Check sheet for the modelled part. Datum: model origin and axes. Units: mm. Face numbers are marked on the shaded views. Coordinates: 2 decimals unless noted, no trailing zeros. Write each loop counter-clockwise with the first axis right and the second up, starting at its lowest first coordinate (ties: lowest second). Pieces come first, ordered by that corner, then holes. Notation, with made-up numbers: (59.25, 89) - (70.25, 89) arc R17 cw to (70.25, 93) - close; hole circle Ø10 at (83.5, 89.5). An arc over 180 degrees is marked (long way). Write each question's results on one line, items separated by ' | '.
from build123d import *

# Parameters (mm, degrees)
SKETCH1_R           = 1.075
SKETCH1_R_2         = 3.5
BOSS_EXTRUDE1_DEPTH = 2.15
SKETCH2_R           = 1.075
BOSS_EXTRUDE2_DEPTH = 2.5


with BuildPart() as part:
    # Sketch1 → Boss-Extrude1 (new body)
    with BuildSketch(Plane(origin=(0, 0, 0), x_dir=(1, 0, 0), z_dir=(0, 1, 0))):
        with BuildLine():
            Line((-30, 19.443650814), (-30, -19.443650814))
            ThreePointArc((-30, -19.443650814), (-30.380602337, -21.357067976), (-31.464466094, -22.97918472))
            Line((-31.464466094, -22.97918472), (-39.242640687, -30.757359313))
            ThreePointArc((-39.242640687, -30.757359313), (-39.242640687, -39.242640687), (-30.757359313, -39.242640687))
            Line((-30.757359313, -39.242640687), (-22.97918472, -31.464466094))
            ThreePointArc((-22.97918472, -31.464466094), (-21.357067976, -30.380602337), (-19.443650814, -30))
            Line((-19.443650814, -30), (19.443650814, -30))
            ThreePointArc((19.443650814, -30), (21.357067976, -30.380602337), (22.97918472, -31.464466094))
            Line((22.97918472, -31.464466094), (30.757359313, -39.242640687))
            ThreePointArc((30.757359313, -39.242640687), (39.242640687, -39.242640687), (39.242640687, -30.757359313))
            Line((39.242640687, -30.757359313), (31.464466094, -22.97918472))
            ThreePointArc((31.464466094, -22.97918472), (30.380602337, -21.357067976), (30, -19.443650814))
            Line((30, -19.443650814), (30, 19.443650814))
            ThreePointArc((30, 19.443650814), (30.380602337, 21.357067976), (31.464466094, 22.97918472))
            Line((31.464466094, 22.97918472), (39.242640687, 30.757359313))
            ThreePointArc((39.242640687, 30.757359313), (39.242640687, 39.242640687), (30.757359313, 39.242640687))
            Line((30.757359313, 39.242640687), (22.97918472, 31.464466094))
            ThreePointArc((22.97918472, 31.464466094), (21.357067976, 30.380602337), (19.443650814, 30))
            Line((19.443650814, 30), (-19.443650814, 30))
            ThreePointArc((-19.443650814, 30), (-21.357067976, 30.380602337), (-22.97918472, 31.464466094))
            Line((-22.97918472, 31.464466094), (-30.757359313, 39.242640687))
            ThreePointArc((-30.757359313, 39.242640687), (-39.242640687, 39.242640687), (-39.242640687, 30.757359313))
            Line((-39.242640687, 30.757359313), (-31.464466094, 22.97918472))
            ThreePointArc((-31.464466094, 22.97918472), (-30.380602337, 21.357067976), (-30, 19.443650814))
        make_face()
        with Locations((-24.245, 24.245)):
            Circle(SKETCH1_R, mode=Mode.SUBTRACT)
        with Locations((24.245, 24.245)):
            Circle(SKETCH1_R, mode=Mode.SUBTRACT)
        with Locations((24.245, -24.245)):
            Circle(SKETCH1_R, mode=Mode.SUBTRACT)
        with Locations((-24.245, -24.245)):
            Circle(SKETCH1_R, mode=Mode.SUBTRACT)
        with Locations((35, -35)):
            Circle(SKETCH1_R_2, mode=Mode.SUBTRACT)
        with Locations((-35, -35)):
            Circle(SKETCH1_R_2, mode=Mode.SUBTRACT)
        with Locations((-35, 35)):
            Circle(SKETCH1_R_2, mode=Mode.SUBTRACT)
        with Locations((35, 35)):
            Circle(SKETCH1_R_2, mode=Mode.SUBTRACT)
        with BuildLine():
            Line((-15, -17.5), (15, -17.5))
            ThreePointArc((15, -17.5), (16.767766953, -16.767766953), (17.5, -15))
            Line((17.5, -15), (17.5, 15))
            ThreePointArc((17.5, 15), (16.767766953, 16.767766953), (15, 17.5))
            Line((15, 17.5), (-15, 17.5))
            ThreePointArc((-15, 17.5), (-16.767766953, 16.767766953), (-17.5, 15))
            Line((-17.5, 15), (-17.5, -15))
            ThreePointArc((-17.5, -15), (-16.767766953, -16.767766953), (-15, -17.5))
        make_face(mode=Mode.SUBTRACT)
    extrude(amount=BOSS_EXTRUDE1_DEPTH)

    # Sketch2 → Boss-Extrude2 (add)
    with BuildSketch(Plane.XZ):
        with BuildLine():
            Line((27.32, -24.245), (27.32, -14.245))
            ThreePointArc((27.32, -14.245), (24.245, -11.17), (21.17, -14.245))
            Line((21.17, -14.245), (21.17, -18.67))
            ThreePointArc((21.17, -18.67), (20.437766953, -20.437766953), (18.67, -21.17))
            Line((18.67, -21.17), (14.245, -21.17))
            ThreePointArc((14.245, -21.17), (11.17, -24.245), (14.245, -27.32))
            Line((14.245, -27.32), (24.245, -27.32))
            ThreePointArc((24.245, -27.32), (26.419353352, -26.419353352), (27.32, -24.245))
        make_face()
        with Locations((24.245, -24.245)):
            Circle(SKETCH2_R, mode=Mode.SUBTRACT)
        with BuildLine():
            Line((-24.245, -27.32), (-14.245, -27.32))
            ThreePointArc((-14.245, -27.32), (-11.17, -24.245), (-14.245, -21.17))
            Line((-14.245, -21.17), (-18.67, -21.17))
            ThreePointArc((-18.67, -21.17), (-20.437766953, -20.437766953), (-21.17, -18.67))
            Line((-21.17, -18.67), (-21.17, -14.245))
            ThreePointArc((-21.17, -14.245), (-24.245, -11.17), (-27.32, -14.245))
            Line((-27.32, -14.245), (-27.32, -24.245))
            ThreePointArc((-27.32, -24.245), (-26.419353352, -26.419353352), (-24.245, -27.32))
        make_face()
        with Locations((-24.245, -24.245)):
            Circle(SKETCH2_R, mode=Mode.SUBTRACT)
        with BuildLine():
            Line((-27.32, 24.245), (-27.32, 14.245))
            ThreePointArc((-27.32, 14.245), (-24.245, 11.17), (-21.17, 14.245))
            Line((-21.17, 14.245), (-21.17, 18.67))
            ThreePointArc((-21.17, 18.67), (-20.437766953, 20.437766953), (-18.67, 21.17))
            Line((-18.67, 21.17), (-14.245, 21.17))
            ThreePointArc((-14.245, 21.17), (-11.17, 24.245), (-14.245, 27.32))
            Line((-14.245, 27.32), (-24.245, 27.32))
            ThreePointArc((-24.245, 27.32), (-26.419353352, 26.419353352), (-27.32, 24.245))
        make_face()
        with Locations((-24.245, 24.245)):
            Circle(SKETCH2_R, mode=Mode.SUBTRACT)
        with BuildLine():
            Line((24.245, 27.32), (14.245, 27.32))
            ThreePointArc((14.245, 27.32), (11.17, 24.245), (14.245, 21.17))
            Line((14.245, 21.17), (18.67, 21.17))
            ThreePointArc((18.67, 21.17), (20.437766953, 20.437766953), (21.17, 18.67))
            Line((21.17, 18.67), (21.17, 14.245))
            ThreePointArc((21.17, 14.245), (24.245, 11.17), (27.32, 14.245))
            Line((27.32, 14.245), (27.32, 24.245))
            ThreePointArc((27.32, 24.245), (26.419353352, 26.419353352), (24.245, 27.32))
        make_face()
        with Locations((24.245, 24.245)):
            Circle(SKETCH2_R, mode=Mode.SUBTRACT)
    extrude(amount=BOSS_EXTRUDE2_DEPTH)


solid = part.part
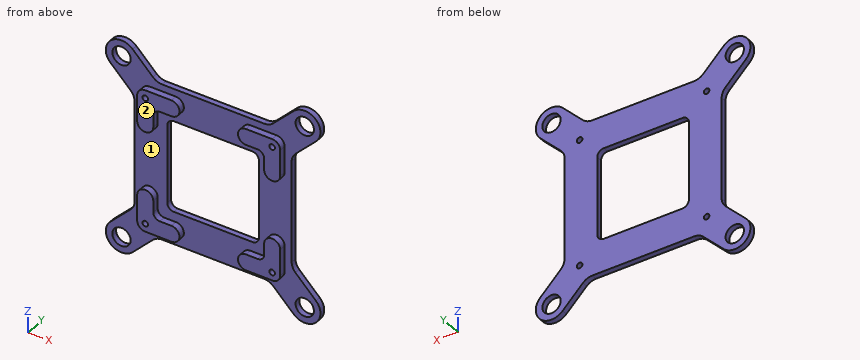
1. Sectioned sample at C-C (y = -1.5). Give the number of separate pieces and of enclosed holes in the cut face, then the cut area to 3 significant figures.
Values follow:
separate pieces: 4 | enclosed holes: 4 | area: 594 mm^2
2. Material ranges on L1, parallel to Z at x = 5, y = 1.4; L2, parallel to X at y = -1.15, z = 14; L3, parallel to Z at x = -23.5, y = -1.9, recorded low to high. Write a range as [from, to].
Values follow:
L1: z = [-30, -17.5], [17.5, 30] | L2: x = [-27.31, -21.18], [21.18, 27.31] | L3: z = [-27.32, -25.02], [-23.47, -11.26], [11.26, 23.47], [25.02, 27.32]
3. Sectioned sample at D-D (x = 36). Record the cut outline in (y, z).
Values follow:
outline: (0, -40.92) - (2.15, -40.92) - (2.15, -38.35) - (0, -38.35) - close; (0, -31.65) - (2.15, -31.65) - (2.15, -27.51) - (0, -27.51) - close; (0, 27.51) - (2.15, 27.51) - (2.15, 31.65) - (0, 31.65) - close; (0, 38.35) - (2.15, 38.35) - (2.15, 40.92) - (0, 40.92) - close
4. Draft check along X on the marked faces 1 and 2. Enter one of: pulls with the +X half, pulls with the -X half, needs draft (parallel to the pull), parting line crosses it, or undercut.
Values follow:
face 1: undercut | face 2: needs draft
5. Sectioned sample at B-B (z = 35). Record the cut outline in (x, y), then the cut area to 3 significant figures.
Values follow:
outline: (-41, 0) - (-38.5, 0) - (-38.5, 2.15) - (-41, 2.15) - close; (-31.5, 0) - (-26.51, 0) - (-26.51, 2.15) - (-31.5, 2.15) - close; (26.51, 0) - (31.5, 0) - (31.5, 2.15) - (26.51, 2.15) - close; (38.5, 0) - (41, 0) - (41, 2.15) - (38.5, 2.15) - close | area: 32.2 mm^2
6. Sectioned sample at A-A (x = 6). Record the cut outline in (y, z).
Values follow:
outline: (0, -30) - (2.15, -30) - (2.15, -17.5) - (0, -17.5) - close; (0, 17.5) - (2.15, 17.5) - (2.15, 30) - (0, 30) - close
7. Go/stop test with flat-tipped pins: pin 1 (1.2 mm diameter, centred on y = -2, z = 17.5, fed in from +X); pin 2 (1 mm diameter, centred on x = 31.5, y = -1.5, fed in from -Z); pin 3 (0.8 mm diameter, centred on x = 17.5, y = -1.5, fed in from +Z); pin 4 (1 mm diameter, centred on y = 0, z = 31.5, fed in from -X). Record where each tip stops, or that it passes through.
Values follow:
pin 1: stops at x = 27.32 | pin 2: passes through | pin 3: stops at z = 27.32 | pin 4: stops at x = -40.2
